```python
from build123d import *

# Parameters (mm, degrees)
SKETCH3_R   = 44.5516
SKETCH3_R_2 = 38.9636
FILLET1_R   = 4.191


with BuildPart() as part:
    # Sketch1 → Revolve1 (revolve)
    with BuildSketch(Plane.XY):
        Polygon((-76.2, -50.2285), (-70.5231, -44.5516), (-70.5231, -38.9636), (-76.2, -44.3865), (-114.3, -44.6405), (-114.3, -50.2285), align=None)
    revolve(axis=Axis((-114.3, 0, 0), (1, 0, 0)))



with BuildPart() as body_2:
    # Sketch2 → Revolve2 (revolve)
    with BuildSketch(Plane.XY):
        Polygon((44.6405, 114.3), (44.3865, 76.2), (38.9636, 70.5231), (44.5516, 70.5231), (50.2285, 76.2), (50.2285, 114.3), align=None)
    revolve(axis=Axis((0, 0, 0), (0, 1, 0)))


with BuildPart() as part_1:
    add(part.part)

    add(body_2.part)  # Sweep1 merges body 2
    # Sweep1: sweep along a path in Sketch4
    with BuildLine(Plane.XY) as sweep1_path:
        ThreePointArc((-70.5231, 0), (-20.65573776, 20.65573776), (0, 70.5231))
    # Sketch3 → Sweep1 (sweep)
    with BuildSketch(Plane(origin=(-70.5231, 0, 0), x_dir=(0, 0, -1), z_dir=(1, 0, 0))):
        Circle(SKETCH3_R)
        Circle(SKETCH3_R_2, mode=Mode.SUBTRACT)
    sweep(path=sweep1_path.line)

    # Fillet1
    fillet1_edges = [part_1.edges().sort_by_distance(p)[0] for p in [
        (-70.5231, 31.502738473, 31.502738473),
        (-31.502738473, 70.5231, 31.502738473),
        (-50.2285, 76.2, 0),
        (-76.2, 50.2285, 0),
    ]]
    fillet(fillet1_edges, radius=FILLET1_R)


solid = part_1.part
```
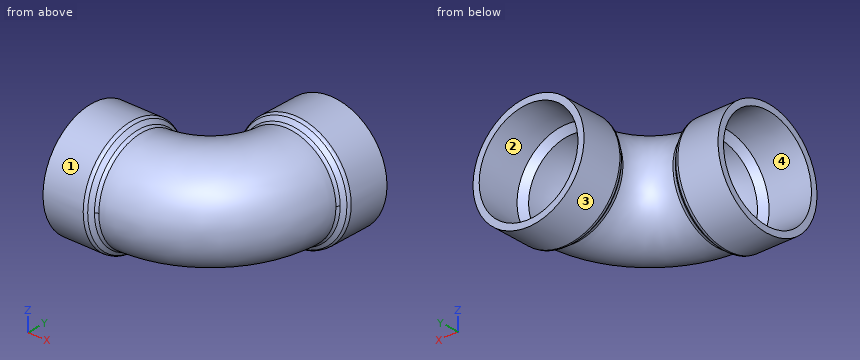
Part model, mm, in its own coordinate system. Face numbers are marked on the shaded views. A direction names the side the tool comes from. Round coordinates to 2 decimals unless told otherwise and drop trailing zeros. Loops run counter-clockwise (first coordinate to the right, second up) from the corner with the lowest first, then second, coordinate; pieces in that order, holes last. Notation, with made-up numbers: (25.5, 8.25) -> (80.5, 8.25) arc R15 ccw to (80.5, 13.25) -> close; hole circle Ø7 at (89.5, 37). An arc over 180 degrees is marked (long way). Use CSV: the item, a comma, the result in double quotes. Start each with the question number.
1) Drop flat-ended pins along their axis: P1, Ø1.5, axis at x = -49, z = -34.5, coming from the +Y side; P2, Ø12, axis at x = 25, y = 51.5, coming from the +Z side; P3, Ø4, axis at x = -2.5, y = 65.5, coming from the -Z side. Give the stop position or say it passes through.
2) Cut at B-B, the plane y = 86. Write the cut outline in (x, z), plus the area to 3 significant figures.
3) Pull direction Z, two halves, no side cores. Call the marked faces 3 and 4: +Z half, -Z half, draft (parallel to the pull), parting line (faces both ways), or undercut.
4) Wall check: L1, parallel to Y at x = -35.5, z = -33; L2, parallel to Z at x = -85.5, y = -16; L3, parallel to Y at x = -48, z = -26. Give the ranges that are in metal, low to high. Write a range as [from, to].
5) Cut at A-A, the plane x = -83. Write the cut outline in (y, z).
6) Which spindle directions (+Z, -Z, +X, -X, +Y, -Y) get a long thin tool onto all of the face, cutting with end or side? Do the marked faces 1 and 2. Say none if no direction does.
Determined:
1,P1,"stops at y = 35.21"
1,P2,"stops at z = 39.36"
1,P3,"stops at z = -44.55"
2,outline,"circle Ø100.46 at (0, 0); hole circle Ø88.9 at (0, 0)"
2,area,"1,720 mm2"
3,face 3,"parting line"
3,face 4,"undercut"
4,L1,"y = [-23.63, -13.73], [35.11, 50], [74.44, 114.3]"
4,L2,"z = [-47.61, -41.47], [41.47, 47.61]"
4,L3,"y = [-33.77, -26.44], [35.66, 44.59]"
5,outline,"circle Ø100.46 at (0, 0); hole circle Ø88.86 at (0, 0)"
6,face 1,"-X"
6,face 2,"+Y"
